Geometry: final body of the model. Coordinates: model frame, mm. Face numbers are marked on the shaded views. Give positions to 0.01 mm unless a question says otherwise; leave off trailing zeros. Order: outer loops, then holes, each group sorted by start corner. A loop starts at its lowest first (then second) coordinate and runs counter-clockwise, first axis right, second up. Notation, with made-up numbers: M -3.75,50.5 L 53.25,50.5 A18 ccw 53.25,55.5 Z; hole C 41,89.5 d3. An arc over 180 degrees is marked long. One line per item, written item: value. Start each with the question number.
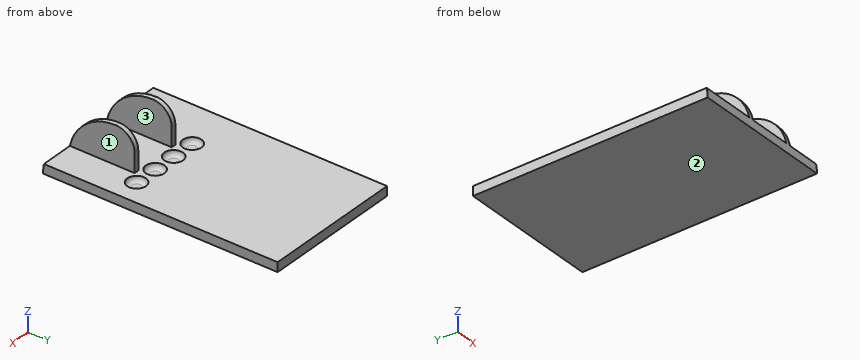
Autodesk Inventor part; units mm, degrees
ref_plane "YZ Plane" through (0, 0, 0) normal (1, 0, 0) x (0, 1, 0)
ref_plane "XZ Plane" through (0, 0, 0) normal (0, 1, 0) x (-1, 0, 0)
ref_plane "XY Plane" through (0, 0, 0) normal (0, 0, 1) x (1, 0, 0)
sketch "Sketch1" plane through (0, 0, 0) normal (0, 0, 1) x (1, 0, 0)
  line L0 (0, 0) -> (15, 0)
  line L1 (15, 0) -> (15, 25)
  line L2 (15, 25) -> (0, 25)
  line L3 (0, 25) -> (0, 0)
  line L4 (0, 7) -> (15, 7) construction
  line L5 (10.94, 7) -> (11.44, 7)
  line L6 (11.44, 7) -> (11.44, 0)
  line L7 (11.44, 0) -> (10.94, 0)
  line L8 (10.94, 0) -> (10.94, 7)
  line L9 (6.36, 7) -> (5.86, 7)
  line L10 (5.86, 7) -> (5.86, 0)
  line L11 (5.86, 0) -> (6.36, 0)
  line L12 (6.36, 0) -> (6.36, 7)
  point P0 (11.19, 7)
  point P1 (6.11, 7)
  dimension "d0" = 15
  dimension "d1" = 25
  dimension "d2" = 18
  dimension "d3" = 3.81
  dimension "d4" = 0.5
  dimension "d5" = 0.5
  dimension "d6" = 5.08
extrude "Extrusion1" add sketch "Sketch1" against normal blind 1
extrude "Extrusion2" add sketch "Sketch1" along normal blind 4 contours L10 L9 L12 L0 | L8 L5 L6 L0
sketch "Sketch2" plane through (0, 0, 0) normal (0, 0, 1) x (1, 0, 0)
  line L0 (0, 7) -> (15, 7) construction
  line L1 (11.44, 7) -> (11.44, 0)
  line L2 (11.44, 0) -> (15, 0)
  line L3 (15, 0) -> (15, 25)
  line L4 (15, 25) -> (0, 25)
  line L5 (0, 25) -> (0, 0)
  line L6 (0, 0) -> (5.86, 0)
  line L7 (5.86, 0) -> (5.86, 7)
  line L8 (5.86, 7) -> (6.36, 7)
  line L9 (6.36, 7) -> (6.36, 0)
  line L10 (6.36, 0) -> (10.94, 0)
  line L11 (10.94, 0) -> (10.94, 7)
  line L12 (10.94, 7) -> (11.44, 7)
  circle A0 centre (12.46, 8) radius 1
  circle A1 centre (9.92, 8) radius 1
  circle A2 centre (7.38, 8) radius 1
  circle A3 centre (4.84, 8) radius 1
  dimension "d11" = 2
  dimension "d12" = 2.54
  dimension "d13" = 1
  dimension "d16" = 2.54
extrude "Extrusion3" cut sketch "Sketch2" against normal blind 0.5 contours A0 | A1 | A2 | A3
fillet "Fillet1" radius 0.5 4 edges at (11.46, 8, -0.5) (8.92, 8, -0.5) (6.38, 8, -0.5) (3.84, 8, -0.5)
fillet "Fillet2" radius 5 2 edges at (6.11, 0, 4) (11.19, 0, 4)
fillet "Fillet3" radius 2 2 edges at (6.11, 7, 4) (11.19, 7, 4)
equation "\"d5\" = d4"
properties part number "mateksys_micro_bec_support"
Q1. Section query C-C on z = -0.25. Return loops of the section in (x, y), and give its area (3 significant figures).
Q2. Section query B-B on z = 2.9. Return loops of the section in (x, y).
Q3. Ray query, line 1 along Z through (x, y) = (9.25, 21.5); line 2 along Y through (x, z) = (2, -0.8). Return the intervals inside material, ascending. Write a range as [from, to].
Q4. Contact query for flat-ended pins moving along their axis: pin 1 (0.8 mm diameter, centred on x = 9.5, y = 8, fed in from +Z); pin 2 (1.2 mm diameter, centred on x = 4.84, y = 8, fed in from +Z); pin 3 (2.5 mm diameter, centred on x = 9.92, y = 8, fed in from +Z). Output: stop coordinate, or through.
Q5. Mould query, pull axis X, two halves, no side actions, for the marked faces 1, 2 and 3. Classes: +X half, -X half, draft (parallel to the pull), parting line (faces both ways), or undercut.
Results below:
1. outline: M 0,0.06 L 15,0.06 L 15,25 L 0,25 Z; hole C 4.84,8 d1.87; hole C 7.38,8 d1.87; hole C 9.92,8 d1.87; hole C 12.46,8 d1.87
1. area: 363 mm2
2. outline: M 5.86,1.87 L 6.36,1.87 L 6.36,6.79 L 5.86,6.79 Z; M 10.94,1.87 L 11.44,1.87 L 11.44,6.79 L 10.94,6.79 Z
3. line 1: [-1, 0]
3. line 2: [0, 25]
4. pin 1: z = -0.38
4. pin 2: z = -0.49
4. pin 3: z = 0
5. face 1: +X half
5. face 2: draft
5. face 3: undercut
